Here's how the part is built. I have some questions about the finished solid (model axes, mm). Face numbers are marked on the shaded views. Round coordinates to 2 decimals unless told otherwise and drop trailing zeros. Order: outer loops, then holes, each group sorted by start corner. A loop starts at its lowest first (then second) coordinate and runs counter-clockwise, first axis right, second up. Notation, with made-up numbers: (-11.75, 77.5) - (0.25, 77.5) arc R16 ccw to (0.25, 87.5) - close; hole circle Ø4 at (-34, -6.5). An arc over 180 degrees is marked (long way). Answer as a JSON object with one key per item and string values.
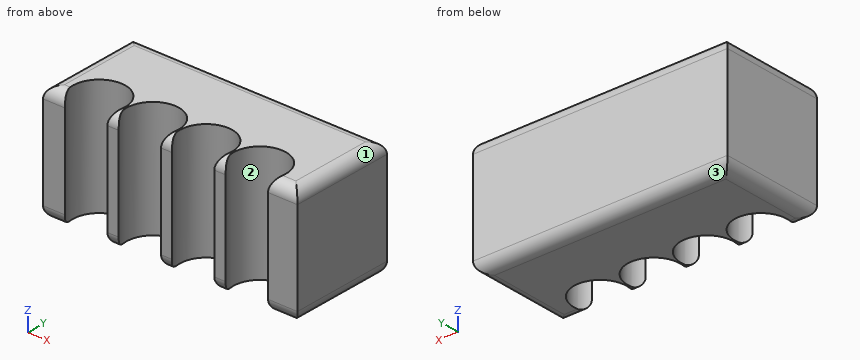
```python
from build123d import *

# Parameters (mm, degrees)
F0_W     = 110
F0_H     = 50
F1_DEPTH = 45
F2_R     = 5
F3_R     = 11.25
F4_DEPTH = 50
F5_DEPTH = 25


with BuildPart() as f1:
    # F0 (on Front) → F1 (new body)
    with BuildSketch(Plane.XZ):
        with Locations((21.923708, -2.648987)):
            Rectangle(F0_W, F0_H)
    extrude(amount=F1_DEPTH)

    # F2
    f2_edges = [f1.edges().sort_by_distance(p)[0] for p in [
        (76.923708, -22.5, 22.351013),
        (-33.076292, -22.5, 22.351013),
        (21.923708, 0, 22.351013),
        (21.923708, -45, 22.351013),
        (-33.076292, -22.5, -27.648987),
        (76.923708, -22.5, -27.648987),
        (21.923708, 0, -27.648987),
        (21.923708, -45, -27.648987),
    ]]
    fillet(f2_edges, radius=F2_R)

    # F3 (on Top) → F4 (cut)
    with BuildSketch(Plane.XY):
        with Locations((-14.420521, -38.467415)):
            Circle(F3_R)
        with Locations((8.798155, -38.467415)):
            Circle(F3_R)
        with Locations((31.823341, -38.467415)):
            Circle(F3_R)
        with Locations((55.042014, -38.467415)):
            Circle(F3_R)
    extrude(amount=-F4_DEPTH, mode=Mode.SUBTRACT)

    # F3 (on Top) → F5 (cut)
    with BuildSketch(Plane.XY):
        with Locations((-14.420521, -38.467415)):
            Circle(F3_R)
        with Locations((8.798155, -38.467415)):
            Circle(F3_R)
        with Locations((31.823341, -38.467415)):
            Circle(F3_R)
        with Locations((55.042014, -38.467415)):
            Circle(F3_R)
    extrude(amount=F5_DEPTH, mode=Mode.SUBTRACT)


solid = f1.part
```
1. Thinking about a two-plate mould opening in X: for the marked faces 1, 2 and 3, which applies, pulls with the +X half, pulls with the -X half, needs draft (parallel to the pull), parting line crosses it, or undercut?
Responses:
{"face 1": "pulls with the +X half", "face 2": "undercut", "face 3": "needs draft"}
2. Imagine slicing it at B-B (z = -12.5). List the corners of the cut face in (x, y) for me, plus the area to 3 significant figures.
Responses:
{"outline": "(-33.08, -45) - (-23.58, -45) arc R11.25 cw (long way) to (-5.26, -45) - (-0.36, -45) arc R11.25 cw (long way) to (17.96, -45) - (22.66, -45) arc R11.25 cw (long way) to (40.98, -45) - (45.88, -45) arc R11.25 cw (long way) to (64.2, -45) - (76.92, -45) - (76.92, 0) - (-33.08, 0) - close", "area": "3,600 mm2"}
3. For P1, Ø8, axis at x = -14.5, z = -13, coming from the -Y side, with a flat end and sliding along its axis, tell me the tip position at first contact or that it passes through.
Responses:
{"P1": "y = -27.98"}
4. If I drill on L1, parallel to X at y = -39.5, z = 3.5; L2, parallel to X at y = -30, z = -25; L3, parallel to Y at x = -17.5, z = -15, over which ranges is the centre line in solid material (lowest first)? Write a range as [from, to].
Responses:
{"L1": "[-33.08, -25.62], [-3.22, -2.4], [20, 20.62], [43.03, 43.84], [66.24, 76.92]", "L2": "[-32.49, -21.83], [-7.01, 1.39], [16.21, 24.42], [39.23, 47.63], [62.45, 76.34]", "L3": "[-27.65, 0]"}
5. Imagine slicing it at A-A (y = -33). List the corners of the cut face in (x, z) for me, plus the area to 3 significant figures.
Responses:
{"outline": "(-33.08, -22.65) arc R5 ccw to (-28.08, -27.65) - (-24.25, -27.65) - (-24.25, 22.35) - (-28.08, 22.35) arc R5 ccw to (-33.08, 17.35) - close; (-4.59, -27.65) - (-1.03, -27.65) - (-1.03, 22.35) - (-4.59, 22.35) - close; (18.63, -27.65) - (21.99, -27.65) - (21.99, 22.35) - (18.63, 22.35) - close; (41.66, -27.65) - (45.21, -27.65) - (45.21, 22.35) - (41.66, 22.35) - close; (64.87, -27.65) - (71.92, -27.65) arc R5 ccw to (76.92, -22.65) - (76.92, 17.35) arc R5 ccw to (71.92, 22.35) - (64.87, 22.35) - close", "area": "1,550 mm2"}
6. Imagine slicing it at D-D (x = -20.5). List the corners of the cut face in (y, z) for me, plus the area to 3 significant figures.
Responses:
{"outline": "(-29, -27.65) - (-5, -27.65) arc R5 ccw to (0, -22.65) - (0, 17.35) arc R5 ccw to (-5, 22.35) - (-29, 22.35) - close", "area": "1,440 mm2"}
7. Imagine slicing it at C-C (x = 8). List the corners of the cut face in (y, z) for me, plus the area to 3 significant figures.
Responses:
{"outline": "(-27.25, -27.65) - (-5, -27.65) arc R5 ccw to (0, -22.65) - (0, 17.35) arc R5 ccw to (-5, 22.35) - (-27.25, 22.35) - close", "area": "1,350 mm2"}
